CAD build for the part. Positions are in the model's coordinates, mm. Coordinates: 2 decimals unless noted, no trailing zeros. Loops run counter-clockwise (first coordinate to the right, second up) from the corner with the lowest first, then second, coordinate; pieces in that order, holes last. Notation, with made-up numbers: (51, 83.25) -> (87, 83.25) arc R18 cw to (87, 104.25) -> close; hole circle Ø10 at (37, 61.25). An arc over 180 degrees is marked (long way). Write item = value, one per line. Start each with the question number.
(1) Band-saw the part on B-B (y = -135). Write the cut outline in (x, z).
(2) Drill centre lines: line 1 (Y direction, x = 0.9, z = -43.75); line 2 (Y direction, x = 1.05, z = -72.5); line 3 (Z direction, x = 2.25, y = -45). Where is each one in solid material? Low to high. Write a range as from..to.
(3) Band-saw the part on A-A (z = -43.75). Write the cut outline in (x, y).
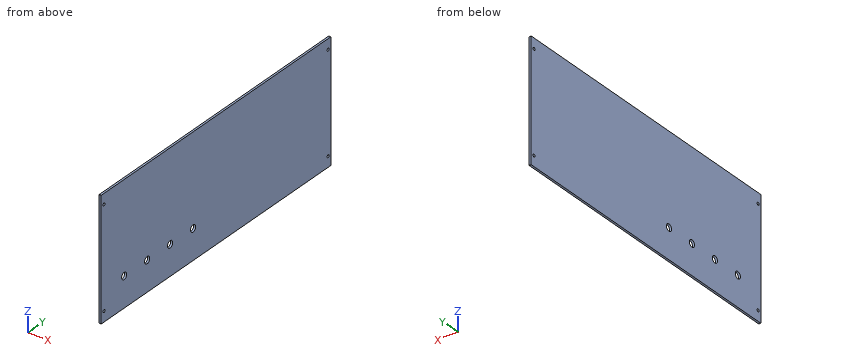
```python
from build123d import *

# Parameters (mm, degrees)
SKETCH1_W           = 175
SKETCH1_H           = 450
SKETCH1_R           = 2
BOSS_EXTRUDE1_DEPTH = 3
SKETCH2_R           = 5
RCA_HOLES_DEPTH     = 242.433738322


with BuildPart() as part:
    # Sketch1 → Boss-Extrude1 (new body)
    with BuildSketch(Plane(origin=(0, 0, 0), x_dir=(0, 0, -1), z_dir=(1, 0, 0))):
        Rectangle(SKETCH1_W, SKETCH1_H)
        with Locations((-72.5, 219.66814109)):
            Circle(SKETCH1_R, mode=Mode.SUBTRACT)
        with Locations((72.5, 219.66814109)):
            Circle(SKETCH1_R, mode=Mode.SUBTRACT)
        with Locations((72.5, -219.66814109)):
            Circle(SKETCH1_R, mode=Mode.SUBTRACT)
        with Locations((-72.5, -219.66814109)):
            Circle(SKETCH1_R, mode=Mode.SUBTRACT)
    extrude(amount=BOSS_EXTRUDE1_DEPTH)

    # Sketch2 → RCA_Holes (cut, through all)
    with BuildSketch(Plane(origin=(0, 0, 0), x_dir=(0, 0, -1), z_dir=(1, 0, 0))):
        with Locations((43.75, -90)):
            Circle(SKETCH2_R)
        with Locations((43.75, -45)):
            Circle(SKETCH2_R)
        with Locations(Location((43.75, -135, 0), (0, 0, 180))):
            Circle(SKETCH2_R)
        with Locations(Location((43.75, -180, 0), (0, 0, 180))):
            Circle(SKETCH2_R)
    extrude(amount=RCA_HOLES_DEPTH, mode=Mode.SUBTRACT)


solid = part.part
```
Findings below:
q1.outline = (0, -87.5) -> (3, -87.5) -> (3, -48.75) -> (0, -48.75) -> close; (0, -38.75) -> (3, -38.75) -> (3, 87.5) -> (0, 87.5) -> close
q2.line_1 = -225..-185, -175..-140, -130..-95, -85..-50, -40..225
q2.line_2 = -225..-221.67, -217.67..217.67, 221.67..225
q2.line_3 = -87.5..-48.75, -38.75..87.5
q3.outline = (0, -225) -> (3, -225) -> (3, -185) -> (0, -185) -> close; (0, -175) -> (3, -175) -> (3, -140) -> (0, -140) -> close; (0, -130) -> (3, -130) -> (3, -95) -> (0, -95) -> close; (0, -85) -> (3, -85) -> (3, -50) -> (0, -50) -> close; (0, -40) -> (3, -40) -> (3, 225) -> (0, 225) -> close
